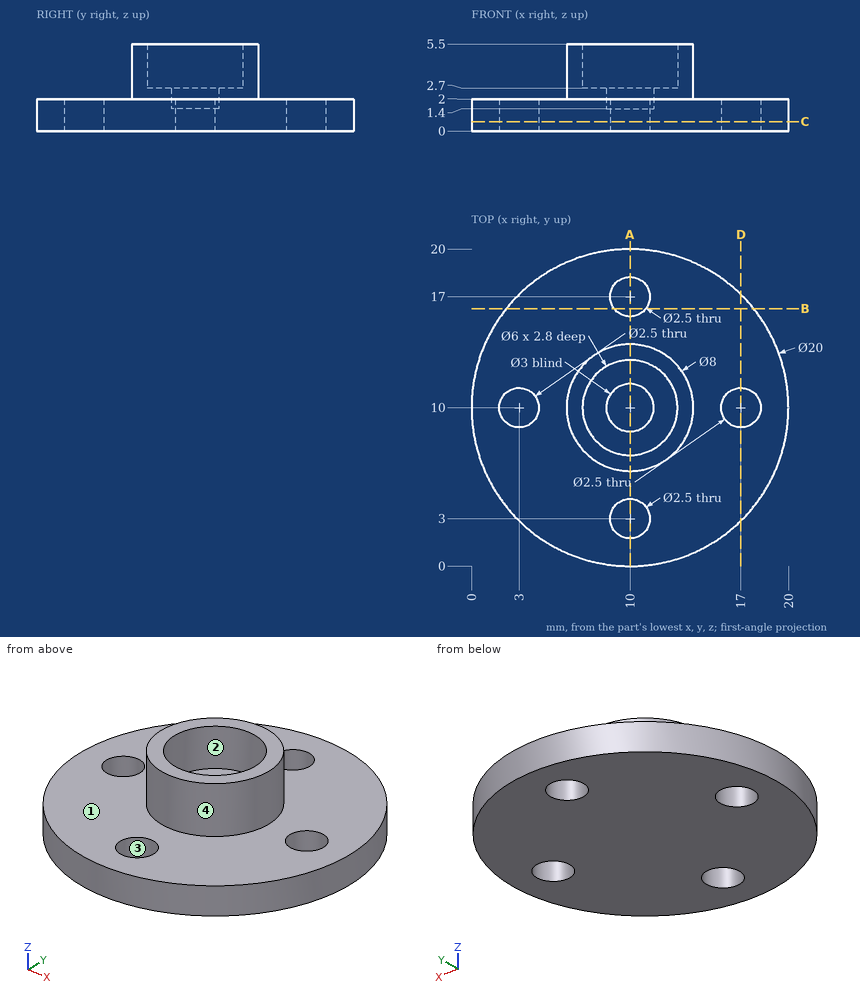
Input: dimensioned drawing with shaded views. Units: mm. Origin: part minimum x, y, z. Coordinates: 2 decimals unless noted, no trailing zeros. Write each loop counter-clockwise with the first axis right and the second up, starting at its lowest first coordinate (ties: lowest second). Pieces come first, ordered by that corner, then holes. Notation, with made-up numbers: M 32,20 L 86,20 A31 cw 86,54 Z; hole C 56.25,57 d2. An arc over 180 degrees is marked long. Answer as a JSON object with one key per item and string values. Group by question number.
(1) Contact query for flat-ended pins moving along their axis: P1, Ø1, axis at x = 17.5, z = 2, coming from the -Y side; P2, Ø2.5, axis at x = 9.5, y = 10, coming from the +Z side; P3, Ø6.5, axis at x = 9, y = 10.5, coming from the +Z side; P4, Ø4, axis at x = 17.5, y = 9, coming from the +Z side. Output: stop coordinate, or through.
(2) Section C-C on z = 0.6. Output: boundary loops of the cut face in (x, y).
(3) Section A-A on x = 10. Output: boundary loops of the cut face in (y, z).
(4) Ray query, line 1 along Y through (x, z) = (10, 1.3); line 2 along Y through (x, z) = (10, 1.8); line 3 along Z through (x, y) = (2.5, 11.5). Return the intervals inside material, ascending. Write a range as [from, to].
(5) Section D-D on x = 17. Output: boundary loops of the cut face in (y, z).
(6) Mould query, pull axis X, two halves, no side actions, for the marked faces 1, 2, 3 and 4. Classes: pulls with the +X half, pulls with the -X half, needs draft (parallel to the pull), parting line crosses it, or undercut.
(7) Section B-B on y = 16.25. Output: boundary loops of the cut face in (x, z).
Result set:
{
 "1": {"P1": "stops at y = 2.86", "P2": "stops at z = 2.7", "P3": "stops at z = 5.5", "P4": "stops at z = 2"},
 "2": {"outline": "C 10,10 d20; hole C 3,10 d2.5; hole C 10,3 d2.5; hole C 10,17 d2.5; hole C 17,10 d2.5"},
 "3": {"outline": "M 0,0 L 1.75,0 L 1.75,2 L 0,2 Z; M 4.25,0 L 15.75,0 L 15.75,2 L 14,2 L 14,5.5 L 13,5.5 L 13,2.7 L 11.5,2.7 L 11.5,1.4 L 8.5,1.4 L 8.5,2.7 L 7,2.7 L 7,5.5 L 6,5.5 L 6,2 L 4.25,2 Z; M 18.25,0 L 20,0 L 20,2 L 18.25,2 Z"},
 "4": {"line 1": "y = [0, 1.75], [4.25, 15.75], [18.25, 20]", "line 2": "y = [0, 1.75], [4.25, 8.5], [11.5, 15.75], [18.25, 20]", "line 3": "z = [0, 2]"},
 "5": {"outline": "M 2.86,0 L 8.75,0 L 8.75,2 L 2.86,2 Z; M 11.25,0 L 17.14,0 L 17.14,2 L 11.25,2 Z"},
 "6": {"face 1": "needs draft", "face 2": "undercut", "face 3": "undercut", "face 4": "parting line crosses it"},
 "7": {"outline": "M 2.19,0 L 9,0 L 9,2 L 2.19,2 Z; M 11,0 L 17.81,0 L 17.81,2 L 11,2 Z"}
}
